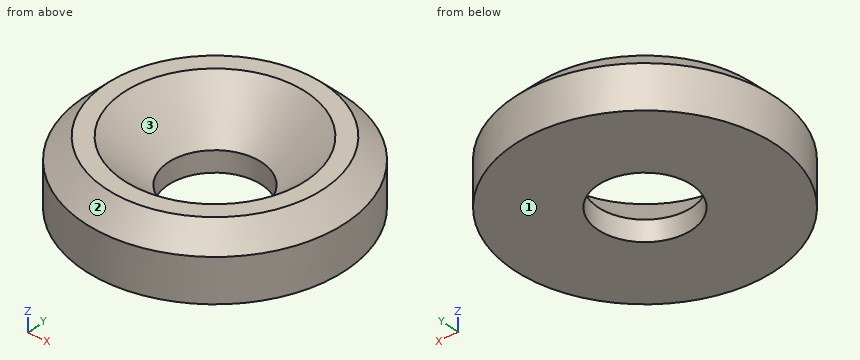
Autodesk Inventor part; units mm, degrees
ref_plane "YZ Plane" through (0, 0, 0) normal (1, 0, 0) x (0, 1, 0)
ref_plane "XZ Plane" through (0, 0, 0) normal (0, 1, 0) x (-1, 0, 0)
ref_plane "XY Plane" through (0, 0, 0) normal (0, 0, 1) x (1, 0, 0)
sketch "Skizze1" plane through (0, 0, 0) normal (0, 0, 1) x (1, 0, 0)
  circle A0 centre (0, 0) radius 6
  dimension "d0" = 12
extrude "Extrusion1" add sketch "Skizze1" along normal blind 3
chamfer "Fasen1" distance 1 angle 45 1 edges at (-6, 0, 3)
sketch "Skizze2" plane through (0, 0, 3) normal (0, 0, 1) x (1, 0, 0)
  circle A0 centre (0, 0) radius 5
hole "Bohrung1" at (0, 0, 3) direction (0, 0, -1) diameter 4.3 depth 3 countersink diameter 8.4 countersink angle 90
properties part number "Druckscheibe" material "Titan"
For this review, take the finished solid that the model builds, in its own axes (mm). Face numbers are marked on the shaded views. Give positions to 0.01 mm unless a question says otherwise; leave off trailing zeros. Order: outer loops, then holes, each group sorted by start corner. A loop starts at its lowest first (then second) coordinate and runs counter-clockwise, first axis right, second up. Notation, with made-up numbers: (70.25, 30) - (80.25, 30) arc R32 cw to (80.25, 61) - close; hole circle Ø4 at (4, 31.25). An arc over 180 degrees is marked (long way). Answer as a JSON object with one key per item and string values. Group by question number.
Item 1: Take a section at C-C on z = 2.7. Give the boundary of the cut face in (x, y), and give its area (3 significant figures).
Item 2: Take a section at A-A on x = 0. Give the boundary of the cut face in (y, z), and give its area (3 significant figures).
Item 3: Take a section at D-D on z = 0.8. Give the boundary of the cut face in (x, y).
Item 4: Draft analysis for pull direction X (two halves, no side actions). For the marked faces 1, 2 and 3, state which applies: pulls with the +X half, pulls with the -X half, needs draft (parallel to the pull), parting line crosses it, or undercut.
Item 5: Wall thickness on line 1 along Y through (x, z) = (0, 0.45); line 2 along X through (y, z) = (2.5, 2.4); line 3 along X through (y, z) = (1.75, 0.6): over which ranges is each line inside the solid? List them lowest first.
Item 6: Clearance check with flat-ended pins moving along their axes: pin 1 Ø7 at (x, y) = (0, 0) entering from +Z; pin 2 Ø1 at (x, z) = (4.5, 1) entering from -Y. State where each tip first meets the part, or that it passes through.
Reported:
{
 "1": {"outline": "circle Ø10.6 at (0, 0); hole circle Ø7.8 at (0, 0)", "area": "40.5 mm^2"},
 "2": {"outline": "(-6, 0) - (-2.15, 0) - (-2.15, 0.95) - (-4.2, 3) - (-5, 3) - (-6, 2) - close; (2.15, 0) - (6, 0) - (6, 2) - (5, 3) - (4.2, 3) - (2.15, 0.95) - close", "area": "17.9 mm^2"},
 "3": {"outline": "circle Ø12 at (0, 0); hole circle Ø4.3 at (0, 0)"},
 "4": {"face 1": "needs draft", "face 2": "parting line crosses it", "face 3": "undercut"},
 "5": {"line 1": "-6 to -2.15, 2.15 to 6", "line 2": "-5.01 to -2.59, 2.59 to 5.01", "line 3": "-5.74 to -1.25, 1.25 to 5.74"},
 "6": {"pin 1": "z = 2.3", "pin 2": "y = -4.47"}
}
